For this review, take the finished solid that the model builds, in its own axes (mm). A direction names the side the tool comes from. Coordinates: 2 decimals unless noted, no trailing zeros. Write each loop counter-clockwise with the first axis right and the second up, starting at its lowest first coordinate (ties: lowest second). Pieces come first, ordered by that corner, then holes.
1) To check wall thickness, follow line 1 along X through (y, z) = (87, 9); line 2 along Y through (x, z) = (-23.5, 8); line 3 along Y through (x, z) = (-3, 6). State the ranges of each line that lie inside material, in increasing order.
2) We need section B-B on y = 70. Write out the cut boundary in (x, z).
3) For faces 1 (the face through (-1, 6, 0)), 2 (the face through (39, -10, 5)), list the 3-axis set-ups (+Z, -Z, +X, -X, +Y, -Y) from which the entire face can be reached by the end or side of a thin tool; tool diameter is ignored.
4) We need section A-A on z = 2. Write out the cut boundary in (x, y), then the cut area to 3 significant figures.
5) Insertion check: P1, Ø3, axis at y = 80, z = 4.5, coming from the +X side; P2, Ø3, axis at x = 41.5, z = 2.5, coming from the +Y side; P3, Ø3, axis at x = 33.5, z = 6, coming from the -Y side. Each pin has a flat end and moves straight along its axis. Give the tip position at first contact, or say it passes through.
6) We need section C-C on x = -36. Write out the cut boundary in (y, z).
from build123d import *

# Parameters (mm, degrees)
BOSS_EXTRU_1_DEPTH      = 10
ENL_V_MAT_EXTRU_1_DEPTH = 100


with BuildPart() as part:
    # Esquisse1 → Boss.-Extru.1 (new body)
    with BuildSketch(Plane.XY):
        Polygon((-50, -105), (50, -105), (50, -10), (27, -10), (27, 105), (-50, 105), align=None)
    extrude(amount=BOSS_EXTRU_1_DEPTH)

    # Esquisse7 → Enlèv. mat.-Extru.1 (cut)
    with BuildSketch(Plane(origin=(50, 0, 0), x_dir=(0, 0, -1), z_dir=(1, 0, 0))):
        Polygon((-10, -105), (0, -105), (0, -95), align=None)
    extrude(amount=-ENL_V_MAT_EXTRU_1_DEPTH, mode=Mode.SUBTRACT)


solid = part.part
Result:
1. line 1: x = -50 to 27
1. line 2: y = -103 to 105
1. line 3: y = -101 to 105
2. outline: (-50, 0) - (27, 0) - (27, 10) - (-50, 10) - close
3. face 1: -Z, +X, -X, +Y, -Y
3. face 2: +Z, -Z, +X, +Y
4. outline: (-50, -97) - (50, -97) - (50, -10) - (27, -10) - (27, 105) - (-50, 105) - close
4. area: 17,600 mm2
5. P1: stops at x = 27
5. P2: stops at y = -10
5. P3: stops at y = -102.5
6. outline: (-105, 10) - (-95, 0) - (105, 0) - (105, 10) - close
